Here's how the part is built. I have some questions about the finished solid (model axes, mm). A direction names the side the tool comes from. Coordinates: 2 decimals unless noted, no trailing zeros. Loops run counter-clockwise (first coordinate to the right, second up) from the corner with the lowest first, then second, coordinate; pieces in that order, holes last. Notation, with made-up numbers: (-27.5, -23) -> (-21.5, -23) arc R23 cw to (-21.5, -14) -> close; hole circle Ø2 at (-31, -2). An arc over 180 degrees is marked (long way). Answer as a JSON object with one key per item and string values. Group by question number.
1) I want a section at A-A (z = 9.5). Write out the boundary of the cut face in (x, y).
2) I want a section at B-B (y = 0). Write out the boundary of the cut face in (x, z), then the cut area to 3 significant figures.
3) I want a section at D-D (z = 15.5). Write out the boundary of the cut face in (x, y).
4) I need wall thicknesses on probe 1 along X at (y, z) = (-30.75, 9.5); probe 2 along Y at (x, z) = (0, 8); probe 3 along Z at (x, y) = (38, -31). Which ranges of each line are inside material? Lowest first, please. Write a range as [from, to].
5) I want a section at C-C (x = 0). Write out the boundary of the cut face in (y, z), then the cut area to 3 significant figures.
6) I'm going to push flat-ended pins straight in: pin 1 (4 mm diameter, centred on y = 12, z = 8.5, fed in from -X); pin 2 (9.5 mm diameter, centred on x = 42.5, z = 11, fed in from +Y); pin 3 (8 mm diameter, centred on y = -20, z = 10.5, fed in from +X). Where does each tip first touch, or does it pass through?
7) Which directions (+Z, -Z, +X, -X, +Y, -Y) give clear straight access to the entire face, cutting with the end or side of a thin tool? Please do faces 1 (the flat face through (28, 2, 9)), 2 (the flat face through (-28, 1, 9)), 3 (the flat face through (1, -13, 19)).
8) If we mould it in two halves opening along Y, with no side actions, what happens to faces 4 (the cylindrical face through (11.923, 3.755, 9.367)), 5 (the flat face through (48, -32, 9)), 6 (the flat face through (1, -40, 9))? For each: +Y half, -Y half, draft (parallel to the pull), parting line (faces both ways), or undercut.
```python
from build123d import *

# Parameters (mm, degrees)
SKETCH_1_R          = 12.5
EXTRUDE_1_DEPTH     = 19
SKETCH_2_R          = 4.5
CUT_EXTRUDE_1_DEPTH = 74.986485252


with BuildPart() as part:
    # 草图1 → 凸台-拉伸1 (new body)
    with BuildSketch(Plane.XY):
        Polygon((-48, -40), (-48, -25), (-28, -25), (-28, 28), (28, 28), (28, -25), (48, -25), (48, -40), align=None)
        Circle(SKETCH_1_R, mode=Mode.SUBTRACT)
    extrude(amount=EXTRUDE_1_DEPTH)

    # 草图2 → 切除-拉伸1 (cut, through all)
    with BuildSketch(Plane(origin=(0, -25, 0), x_dir=(1, 0, 0), z_dir=(0, 1, 0))):
        with Locations(Location((-38, -9.5, 0), (0, 0, 270))):
            Circle(SKETCH_2_R)
        with Locations(Location((38, -9.5, 0), (0, 0, 90))):
            Circle(SKETCH_2_R)
    extrude(amount=-CUT_EXTRUDE_1_DEPTH, mode=Mode.SUBTRACT)


solid = part.part
```
Determined:
{
 "1": {"outline": "(-48, -40) -> (-42.5, -40) -> (-42.5, -25) -> (-48, -25) -> close; (-33.5, -40) -> (33.5, -40) -> (33.5, -25) -> (28, -25) -> (28, 28) -> (-28, 28) -> (-28, -25) -> (-33.5, -25) -> close; (42.5, -40) -> (48, -40) -> (48, -25) -> (42.5, -25) -> close; hole circle Ø25 at (0, 0)"},
 "2": {"outline": "(-28, 0) -> (-12.5, 0) -> (-12.5, 19) -> (-28, 19) -> close; (12.5, 0) -> (28, 0) -> (28, 19) -> (12.5, 19) -> close", "area": "589 mm^2"},
 "3": {"outline": "(-48, -40) -> (48, -40) -> (48, -25) -> (28, -25) -> (28, 28) -> (-28, 28) -> (-28, -25) -> (-48, -25) -> close; hole circle Ø25 at (0, 0)"},
 "4": {"probe 1": "[-48, -42.5], [-33.5, 33.5], [42.5, 48]", "probe 2": "[-40, -12.5], [12.5, 28]", "probe 3": "[0, 5], [14, 19]"},
 "5": {"outline": "(-40, 0) -> (-12.5, 0) -> (-12.5, 19) -> (-40, 19) -> close; (12.5, 0) -> (28, 0) -> (28, 19) -> (12.5, 19) -> close", "area": "817 mm^2"},
 "6": {"pin 1": "x = -28", "pin 2": "y = -25", "pin 3": "x = 28"},
 "7": {"face 1": "+Z, -Z, +X, +Y", "face 2": "+Z, -Z, -X, +Y", "face 3": "+Z, +X, -X, +Y, -Y"},
 "8": {"face 4": "undercut", "face 5": "draft", "face 6": "-Y half"}
}
